The model under review builds one solid part; all positions refer to its coordinate system, in mm. Face numbers are marked on the shaded views. A direction names the side the tool comes from. Give positions to 0.01 mm unless a question says otherwise; leave off trailing zeros. Order: outer loops, then holes, each group sorted by start corner. A loop starts at its lowest first (then second) coordinate and runs counter-clockwise, first axis right, second up. Notation, with made-up numbers: M -20.75,86 L 6.25,86 A24 ccw 6.25,100 Z; hole C 85.5,-17.75 d5. An arc over 180 degrees is marked long. One line per question, with ' | ' between items. Start each with the question number.
1. We need section A-A on y = 22. Write out the cut boundary in (x, z) (3 decimals), then the cut area to 3 significant figures.
2. We need section D-D on y = 42. Write out the cut boundary in (x, z) (3 decimals).
3. We need section B-B on z = 6. Write out the cut boundary in (x, y) (3 decimals).
4. Wall thickness on L1, parallel to Z at x = -5, y = -28 (3 decimals); L2, parallel to Y at x = 30, z = 33; L3, parallel to Z at x = 74.5, y = -17.5: over which ranges is each line inside the solid? List them lowest first.
5. For the marked faces 1, 2, 3 and 4, list the 3-axis set-ups (+Z, -Z, +X, -X, +Y, -Y) from which the entire face can be reached by the end or side of a thin tool; tool diameter is ignored.
6. Insertion check: P1, Ø5, axis at y = -28.5, z = 16, coming from the +X side; P2, Ø14, axis at y = -14, z = 19, coming from the -X side; P3, Ø5, axis at y = 12.5, z = 18, coming from the -X side (3 decimals); P4, Ø10, axis at y = -21, z = 8.5, coming from the +X side (3 decimals). Each pin has a flat end and moves straight along its axis. Give the tip position at first contact, or say it passes through.
7. We need section C-C on x = 75. Write out the cut boundary in (y, z).
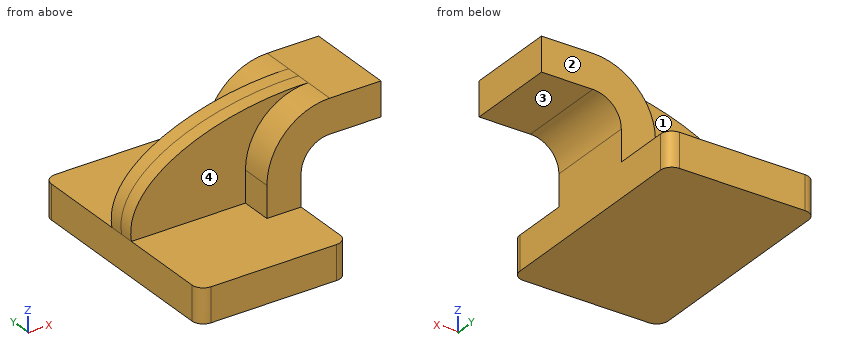
```python
from build123d import *

# Parameters (mm, degrees)
F1_DEPTH = 63.5
F0_W     = 25.4
F0_H     = 19.05
F2_DEPTH = 25.4
F3_DEPTH = 7.9375
F4_R     = 6.35


with BuildPart() as f1:
    # F0 (on Front) → F1 (new body, symmetric)
    with BuildSketch(Plane.XZ):
        Polygon((41.275, -9.525), (41.275, 9.525), (22.225, 9.525), (-41.275, 9.525), (-41.275, -9.525), align=None)
    extrude(amount=F1_DEPTH, both=True)

    # F0 (on Front) → F2 (join, symmetric)
    with BuildSketch(Plane.XZ):
        with BuildLine():
            Line((22.225, 9.525), (41.275, 9.525))
            Line((41.275, 9.525), (41.275, 27.0002))
            ThreePointArc((41.275, 27.0002), (45.92468, 38.22552), (57.15, 42.8752))
            Line((57.15, 42.8752), (60.325, 42.8752))
            Line((60.325, 42.8752), (60.325, 61.9252))
            Line((60.325, 61.9252), (57.15, 61.9252))
            ThreePointArc((57.15, 61.9252), (32.454296, 51.695904), (22.225, 27.0002))
            Line((22.225, 27.0002), (22.225, 9.525))
        make_face()
        with Locations((73.025, 52.4002)):
            Rectangle(F0_W, F0_H)
    extrude(amount=F2_DEPTH, both=True)

    # F0 (on Front) → F3 (join, symmetric)
    with BuildSketch(Plane.XZ):
        with BuildLine():
            Line((-41.275, 9.525), (22.225, 9.525))
            Line((22.225, 9.525), (22.225, 27.0002))
            ThreePointArc((22.225, 27.0002), (32.454296, 51.695904), (57.15, 61.9252))
            add(Edge.make_bspline(
                [(-41.275, 9.525), (-46.898041, 42.469062), (7.599939, 63.057207), (57.15, 61.9252)],
                knots=[0, 0, 0, 0, 111.504536, 111.504536, 111.504536, 111.504536], degree=3))
        make_face()
    extrude(amount=F3_DEPTH, both=True)

    # F4
    f4_edges = [f1.edges().sort_by_distance(p)[0] for p in [
        (41.275, -63.5, 0),
        (-41.275, -63.5, 0),
        (41.275, 63.5, 0),
        (-41.275, 63.5, 0),
    ]]
    fillet(f4_edges, radius=F4_R)


solid = f1.part
```
Entries:
1) outline: M -41.275,-9.525 L 41.275,-9.525 L 41.275,27 A15.875 cw 57.15,42.875 L 85.725,42.875 L 85.725,61.925 L 57.15,61.925 A34.925 ccw 22.225,27 L 22.225,9.525 L -41.275,9.525 Z | area: 3,210 mm^2
2) outline: M -41.275,-9.525 L 41.275,-9.525 L 41.275,9.525 L -41.275,9.525 Z
3) outline: M -41.275,-57.15 A6.35 ccw -34.925,-63.5 L 34.925,-63.5 A6.35 ccw 41.275,-57.15 L 41.275,57.15 A6.35 ccw 34.925,63.5 L -34.925,63.5 A6.35 ccw -41.275,57.15 Z
4) L1: z = -9.525 to 9.525 | L2: y = -25.4 to 25.4 | L3: z = 42.88 to 61.93
5) face 1: +Z, -X, +Y | face 2: +Z, +X, -X, +Y | face 3: -Z, +X, +Y, -Y | face 4: +Z, -X, -Y
6) P1: passes through | P2: stops at x = -41.64 | P3: stops at x = 22.225 | P4: stops at x = 41.275
7) outline: M -25.4,42.88 L 25.4,42.88 L 25.4,61.93 L -25.4,61.93 Z
